from build123d import *

# Parameters (mm, degrees)
F2_W     = 128.6
F2_H     = 128.6
F2_W_2   = 125
F2_H_2   = 125
F3_DEPTH = 36
F4_DEPTH = 1.8
F5_W     = 125
F5_H     = 1.8
F6_DEPTH = 25


with BuildPart() as f3:
    # F2 (on Top) → F3 (new body)
    with BuildSketch(Plane.XY):
        Rectangle(F2_W, F2_H)
        Rectangle(F2_W_2, F2_H_2, mode=Mode.SUBTRACT)
    extrude(amount=F3_DEPTH)

    # F2 (on Top) → F4 (join)
    with BuildSketch(Plane.XY):
        Rectangle(F2_W, F2_H)
        Rectangle(F2_W_2, F2_H_2, mode=Mode.SUBTRACT)
        Rectangle(F2_W_2, F2_H_2)
    extrude(amount=-F4_DEPTH)

    # F5 (on face) → F6 (cut)
    with BuildSketch(Plane.XY.offset(36)):
        with Locations((0, 63.4)):
            Rectangle(F5_W, F5_H)
    extrude(amount=-F6_DEPTH, mode=Mode.SUBTRACT)


solid = f3.part
Could you check a few things on this model? Use its own coordinates, in mm. A direction names the side the tool comes from. Give positions to 0.01 mm unless a question says otherwise; leave off trailing zeros. Order: outer loops, then holes, each group sorted by start corner. A loop starts at its lowest first (then second) coordinate and runs counter-clockwise, first axis right, second up.
Item 1: I need wall thicknesses on line 1 (Y direction, x = 57, z = 10.5); line 2 (Y direction, x = 16, z = 28). Which ranges of each line are inside material? Lowest first, please.
Item 2: For faces 1 (the face through (0, 64.3, 6)), 2 (the face through (-1, 62.5, 5)), which set-ups out of +Z, -Z, +X, -X, +Y, -Y let a thin tool reach every point of the face, with its end or its side?
Item 3: If we section it at A-A, the plane x = -20.5: Write out the boundary of the cut face in (y, z), plus the area to 3 significant figures.
Item 4: If we mould it in two halves opening along X, with no side actions, what happens to faces 3 (the face through (-64.3, -1, 17)), 4 (the face through (-62.5, 0, 18)), 5 (the face through (-1, -64.3, 17))? For each: pulls with the +X half, pulls with the -X half, needs draft (parallel to the pull), parting line crosses it, or undercut.
Item 5: If we section it at C-C, the plane y = -33.5: Write out the boundary of the cut face in (x, z), plus the area to 3 significant figures.
Item 6: I'm going to push flat-ended pins straight in: pin 1 (0.5 mm diameter, centred on x = 26.5, y = 63.5, fed in from +Z); pin 2 (1 mm diameter, centred on x = 3.5, z = 19.5, fed in from +Y); pin 3 (1.5 mm diameter, centred on x = -23, y = 40.5, fed in from +Z). Where does each tip first touch, or does it pass through?
Item 7: If we section it at B-B, the plane z = 4.5: Write out the boundary of the cut face in (x, y), plus the area to 3 significant figures.
Values:
1. line 1: y = -64.3 to -62.5, 62.5 to 64.3
1. line 2: y = -64.3 to -62.5
2. face 1: +Z, -Z, +X, -X, +Y
2. face 2: +Z
3. outline: (-64.3, -1.8) - (64.3, -1.8) - (64.3, 11) - (62.5, 11) - (62.5, 0) - (-62.5, 0) - (-62.5, 36) - (-64.3, 36) - close
3. area: 316 mm2
4. face 3: pulls with the -X half
4. face 4: undercut
4. face 5: needs draft
5. outline: (-64.3, -1.8) - (64.3, -1.8) - (64.3, 36) - (62.5, 36) - (62.5, 0) - (-62.5, 0) - (-62.5, 36) - (-64.3, 36) - close
5. area: 361 mm2
6. pin 1: stops at z = 11
6. pin 2: stops at y = -62.5
6. pin 3: stops at z = 0
7. outline: (-64.3, -64.3) - (64.3, -64.3) - (64.3, 64.3) - (-64.3, 64.3) - close; hole (-62.5, -62.5) - (62.5, -62.5) - (62.5, 62.5) - (-62.5, 62.5) - close
7. area: 913 mm2
